```python
from build123d import *

# Parameters (mm, degrees)
F1_W      = 24
F1_H      = 30
F2_DEPTH  = 8
F3_T      = -1.5
F4_W      = 3
F4_H      = 12
F5_DEPTH  = 5
F6_W      = 8
F6_H      = 25
F7_DEPTH  = 30
F8_W      = 3.5
F8_H      = 1.5
F9_DEPTH  = 4
F10_SIZE  = 0.8
F11_R     = 1.5
F12_DEPTH = 25
F13_R     = 0.5
F14_SIZE  = 0.5
F15_R     = 0.5
F16_DEPTH = 5
F17_SIZE  = 1.49999


# Not quite as in the source:
# - a fillet or chamfer is up to 0.001 mm smaller than in the source, because OpenCascade refuses the exact size


with BuildPart() as f2:
    # F1 (on Right) → F2 (new body)
    with BuildSketch(Plane.YZ):
        with Locations((-10, -15)):
            Rectangle(F1_W, F1_H)
    extrude(amount=-F2_DEPTH)

    # F3
    f3_openings = [f2.faces().sort_by_distance(p)[0] for p in [
        (0, -10, -15),
    ]]
    offset(amount=F3_T, openings=f3_openings)

    # F4 (on Top) → F5 (cut)
    with BuildSketch(Plane.XY):
        with Locations((0, -10)):
            Rectangle(F4_W, F4_H)
        with Locations((-4.5, -10)):
            Rectangle(F4_W, F4_H)
    extrude(amount=-F5_DEPTH, mode=Mode.SUBTRACT)

    # F6 (on face) → F7 (cut)
    with BuildSketch(Plane.XZ.offset(22)):
        with Locations((-1.8903282698, -15)):
            Rectangle(F6_W, F6_H)
    extrude(amount=-F7_DEPTH, mode=Mode.SUBTRACT)

    # F8 (on Right) → F9 (join, symmetric)
    with BuildSketch(Plane.YZ):
        with Locations((-18.25, -2.25)):
            Rectangle(F8_W, F8_H)
        with Locations((-1.75, -27.75)):
            Rectangle(F8_W, F8_H)
    extrude(amount=F9_DEPTH, both=True)

    # F10
    f10_edges = [f2.edges().sort_by_distance(p)[0] for p in [
        (4, -18.25, -1.5),
        (4, -1.75, -27),
    ]]
    chamfer(f10_edges, length=F10_SIZE)

    # F11 (on Right) → F12 (cut)
    with BuildSketch(Plane.YZ):
        with Locations((-10, -17)):
            Circle(F11_R)
    extrude(amount=-F12_DEPTH, mode=Mode.SUBTRACT)

    # F13
    f13_edges = [f2.edges().sort_by_distance(p)[0] for p in [
        (-4, 2, 0),
        (-8, 2, -15),
        (-4, -22, 0),
        (-4, -22, -30),
        (-4, 2, -30),
        (-8, -10, 0),
        (-8, -22, -15),
        (-8, -10, -30),
    ]]
    fillet(f13_edges, radius=F13_R)

    # F14
    f14_edges = [f2.edges().sort_by_distance(p)[0] for p in [
        (-5.890328, 2, -15),
        (-2.945164, 2, -2.5),
        (-2.945164, 2, -27.5),
        (-2.945164, -22, -2.5),
        (-5.890328, -22, -15),
        (-2.945164, -22, -27.5),
    ]]
    chamfer(f14_edges, length=F14_SIZE)

    # F15 (on face) → F16 (join)
    with BuildSketch(Plane.YZ.offset(-6.5)):
        with Locations((-13, -4.5)):
            Circle(F15_R)
        with Locations((-7, -4.5)):
            Circle(F15_R)
    extrude(amount=F16_DEPTH)

    # F17 (size 1.5 in the source; OpenCascade refuses exactly that, so slightly less here)
    f17_edges = [f2.edges().sort_by_distance(p)[0] for p in [
        (-4, -18.25, -3),
        (-4, -1.75, -27),
    ]]
    chamfer(f17_edges, length=F17_SIZE)


solid = f2.part
```
Verification items for the finished model (mm, model axes). A direction names the side the tool comes from. Give positions to 0.01 mm unless a question says otherwise; leave off trailing zeros. Write each loop counter-clockwise with the first axis right and the second up, starting at its lowest first coordinate (ties: lowest second). Pieces come first, ordered by that corner, then holes. Notation, with made-up numbers: M 70,39.25 L 120,39.25 A17 ccw 120,57.25 Z; hole C -29.75,-23 d3. An arc over 180 degrees is marked long. One line per question, with ' | ' between items.
1) Mould release check, pull along Y, two halves, no side actions. Record for faces 1 (the flat face through (3.6, -1.8, -27.4)), 2 (the cylindrical face through (-4, -7, -4)), 3 (the flat face through (-7, 2, -15)), 4 (the flat face through (-3.2, -1.8, -27.7)): released by +Y, released by -Y, zero draft, split by the parting line, or undercut.
Result:
face 1: zero draft | face 2: undercut | face 3: released by +Y | face 4: undercut
2) Set-up check for faces 5 (the flat face through (-3.2, -18.3, -2.3)), 6 (the flat face through (-3, -21, -2.5)), 7 (the flat face through (-5, -4, -1)), 8 (the cylindrical face through (-4, -13, -4)): record each of +Z, -Z, +X, -X, +Y, -Y from which the full face is reachable in a straight line by a thin tool's end or side.
Result:
face 5: none | face 6: +X, -Y | face 7: +Z | face 8: +X
3) Section check A-A on x = -4.5. State how many separate pieces and enclosed holes the cut face has, plus the area to 3 significant figures.
Result:
separate pieces: 5 | enclosed holes: 0 | area: 60.9 mm2
4) Section check C-C on z = -17. Enter the section's corners in (x, y).
Result:
outline: M -8,-21.5 A0.5 ccw -7.5,-22 L -6.39,-22 L -5.89,-21.5 L -5.89,-20.5 L -6.5,-20.5 L -6.5,-11.5 L -8,-11.5 Z; M -8,-8.5 L -6.5,-8.5 L -6.5,0.5 L -5.89,0.5 L -5.89,1.5 L -6.39,2 L -7.5,2 A0.5 ccw -8,1.5 Z
5) Thickness scan on line 1 along Z through (x, y) = (-7.5, -10); line 2 along X through (y, z) = (-15.75, -20.25); line 3 along Y through (x, z) = (1.25, -2.25). Record the ranges inside material, lowest first. Write a range as [from, to].
Result:
line 1: z = [-30, -18.5], [-15.5, 0] | line 2: x = [-8, -6.5] | line 3: y = [-20, -16.5]
6) Section check B-B on y = -5.25. Enter the section's corners in (x, z).
Result:
outline: M -8,-29.5 A0.5 ccw -7.5,-30 L 0,-30 L 0,-28.5 L -6.5,-28.5 L -6.5,-1.5 L -6,-1.5 L -6,0 L -7.5,0 A0.5 ccw -8,-0.5 Z; M -3,-1.5 L -1.5,-1.5 L -1.5,0 L -3,0 Z
7) Gauge pin test, flat ends, axial feed: pin 1 Ø1.5 at (y, z) = (-9.5, -20.5) entering from +X; pin 2 Ø3 at (y, z) = (-7.5, -28.5) entering from +X; pin 3 Ø1 at (x, y) = (2, -18) entering from -Z. Record the tip position at first contact, or that the pin passes through.
Result:
pin 1: stops at x = -6.5 | pin 2: stops at x = 0 | pin 3: stops at z = -3
